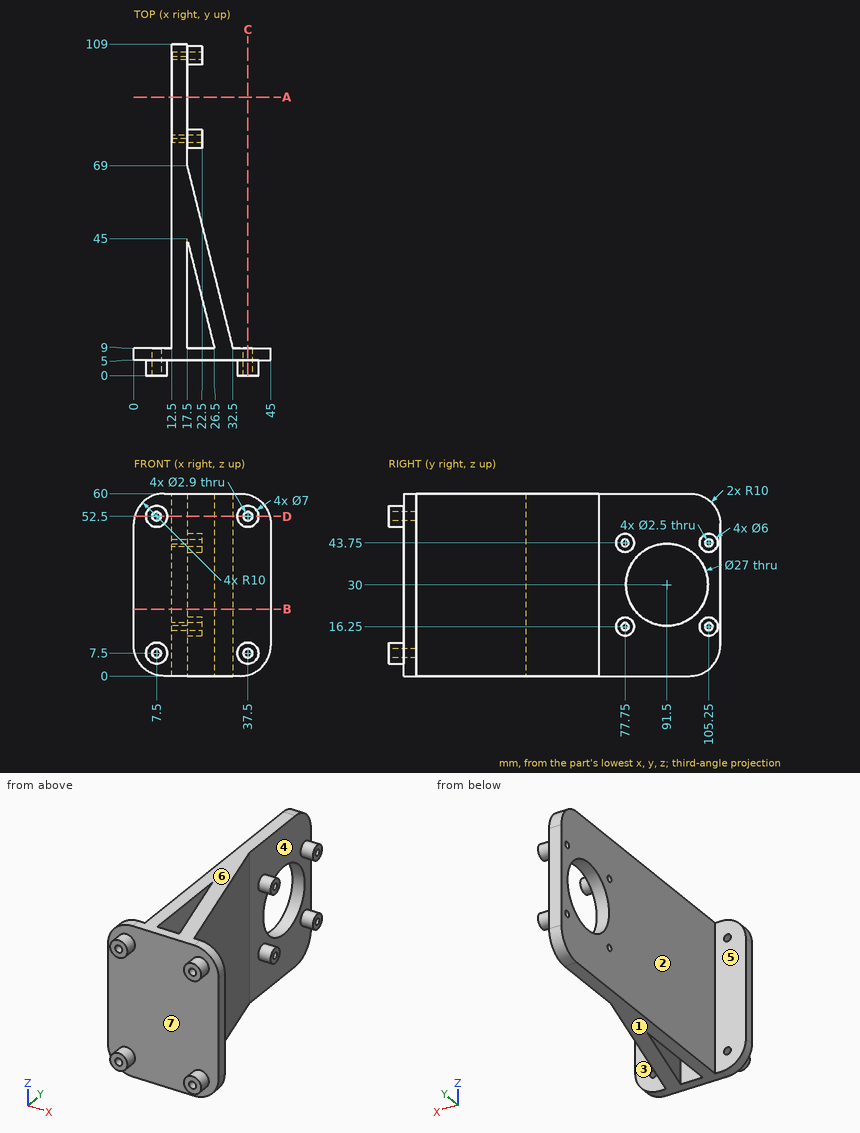
Here's the drawing with two shaded views (mm, measured from the low corner). I have some questions. A direction names the side the tool comes from. Coordinates: 2 decimals unless noted, no trailing zeros. Write each loop counter-clockwise with the first axis right and the second up, starting at its lowest first coordinate (ties: lowest second). Pieces come first, ordered by that corner, then holes.
Item 1: I want a section at D-D on z = 52.5. Write out the boundary of the cut face in (x, y).
Item 2: I want a section at A-A on y = 91.5. Write out the boundary of the cut face in (x, z).
Item 3: If we mould it in two halves opening along Y, with no side actions, what happens to the marked faces 4, 5, 6 and 7? For each: +Y half, -Y half, draft (parallel to the pull), parting line (faces both ways), or undercut.
Item 4: I want a section at C-C on x = 37.5. Write out the boundary of the cut face in (y, z), and give its area (3 significant figures).
Item 5: On a 3-axis mill with a long thin cutter (end or side, diameter ignored), from which of +Z, -Z, +X, -X, +Y, -Y can I reach the whole of each face in a straight line? I mean the marked faces 1, 2 and 3. Say none if no direction works.
Item 6: Will these pins go through, and if not, where does the flat tip stop? pin 1 (4 mm diameter, centred on y = 66, z = 43.5, fed in from -X); pin 2 (3 mm diameter, centred on x = 19, z = 41, fed in from -Y); pin 3 (3.5 mm diameter, centred on x = 7.5, z = 52.5, fed in from +Y); pin 4 (8 mm diameter, centred on x = 10, y = 79, fed in from +Z).
Item 7: If I drill on line 1 (X direction, y = 4.75, z = 52.5); line 2 (Z direction, x = 17.75, y = 77.75); line 3 (Z direction, x = 14.05, y = 91.5), over which ranges is the centre line in solid material (lowest first)?
Item 8: I want a section at B-B on z = 22. Write out the boundary of the cut face in (x, y), and give its area (3 significant figures).
Findings below:
1. outline: (0.32, 5) - (4, 5) - (4, 0) - (6.05, 0) - (6.05, 9) - (0.32, 9) - close; (8.95, 0) - (11, 0) - (11, 5) - (34, 5) - (34, 0) - (36.05, 0) - (36.05, 9) - (32.5, 9) - (17.5, 69) - (17.5, 108.68) - (12.5, 108.68) - (12.5, 9) - (8.95, 9) - close; (38.95, 0) - (41, 0) - (41, 5) - (44.68, 5) - (44.68, 9) - (38.95, 9) - close; hole (17.5, 9) - (26.5, 9) - (17.5, 45) - close
2. outline: (12.5, 0) - (17.5, 0) - (17.5, 16.5) - (12.5, 16.5) - close; (12.5, 43.5) - (17.5, 43.5) - (17.5, 60) - (12.5, 60) - close
3. face 4: undercut
3. face 5: +Y half
3. face 6: draft
3. face 7: -Y half
4. outline: (0, 4) - (5, 4) - (5, 0.32) - (9, 0.32) - (9, 6.05) - (0, 6.05) - close; (0, 8.95) - (9, 8.95) - (9, 51.05) - (0, 51.05) - (0, 49) - (5, 49) - (5, 11) - (0, 11) - close; (0, 53.95) - (9, 53.95) - (9, 59.68) - (5, 59.68) - (5, 56) - (0, 56) - close
4. area: 255 mm2
5. face 1: -Z, +X, -X, +Y, -Y
5. face 2: +Z, -Z, -X, +Y
5. face 3: +Z, -Z, +X, +Y
6. pin 1: stops at x = 12.5
6. pin 2: stops at y = 5
6. pin 3: stops at y = 9
6. pin 4: stops at z = 60
7. line 1: x = 4 to 6.05, 8.95 to 11, 34 to 36.05, 38.95 to 41
7. line 2: z = 13.25 to 15, 17.5 to 19.25, 40.75 to 42.5, 45 to 46.75
7. line 3: z = 0 to 16.5, 43.5 to 60
8. outline: (0, 5) - (45, 5) - (45, 9) - (32.5, 9) - (17.5, 69) - (17.5, 80.63) - (12.5, 80.63) - (12.5, 9) - (0, 9) - close; (12.5, 102.37) - (17.5, 102.37) - (17.5, 109) - (12.5, 109) - close; hole (17.5, 9) - (26.5, 9) - (17.5, 45) - close
8. area: 859 mm2
